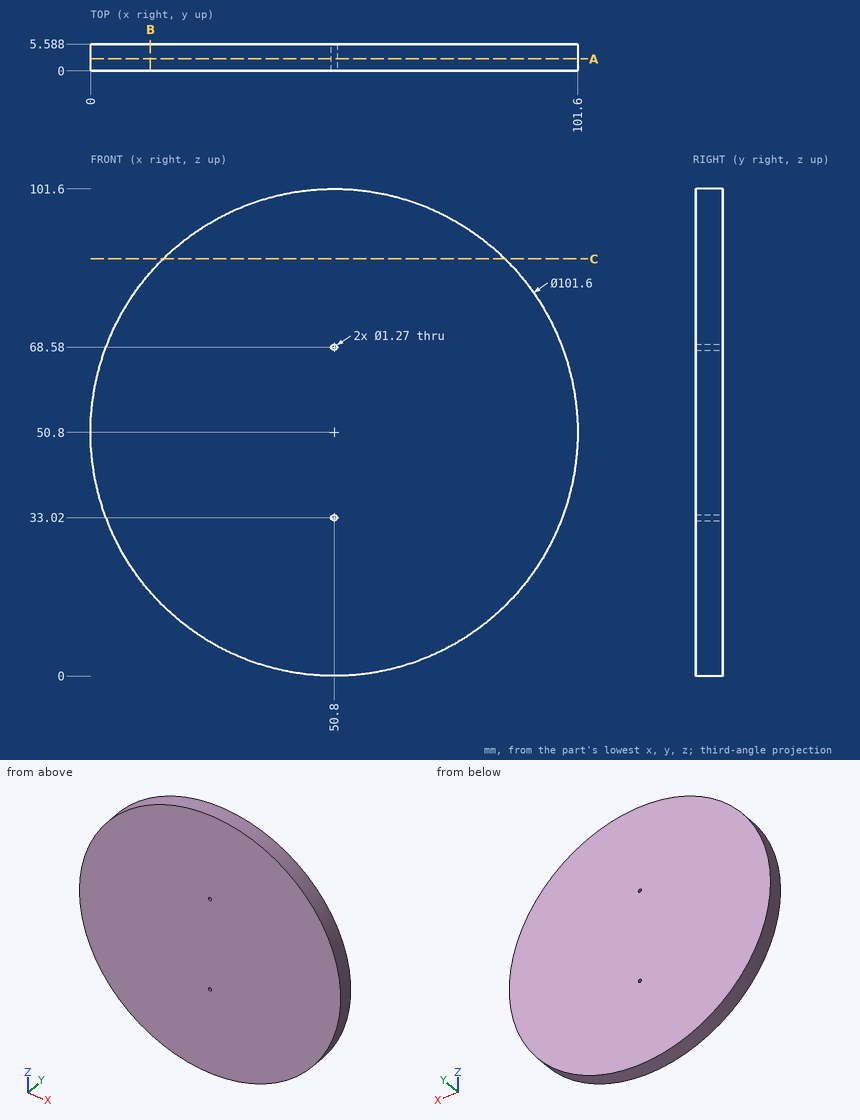
Design review of the part shown in the three views and the two pictorial views. Dimensions are in mm from the part's minimum x, y and z. Give positions to 0.01 mm unless a question says otherwise; leave off trailing zeros. Write each loop counter-clockwise with the first axis right and the second up, starting at its lowest first coordinate (ties: lowest second). Pieces come first, ordered by that corner, then holes.
(1) Wall thickness on line 1 along Z through (x, y) = (50.8, 2.95) (3 decimals); line 2 along X through (y, z) = (2.55, 68.58) (3 decimals); line 3 along Z through (x, y) = (48.5, 2.85): over which ranges is each line inside the solid? List them lowest first.
Checked values:
line 1: z = 0 to 32.385, 33.655 to 67.945, 69.215 to 101.6
line 2: x = 3.213 to 50.165, 51.435 to 98.387
line 3: z = 0.05 to 101.55
(2) Clearance check with flat-ended pins moving along their axes: pin 1 Ø3 at (y, z) = (3, 69) entering from +X; pin 2 Ø3 at (y, z) = (3, 47) entering from -X; pin 3 Ø3 at (x, y) = (44.5, 2) entering from +Z. State where each tip first meets the part, or that it passes through.
Checked values:
pin 1: stops at x = 98.78
pin 2: stops at x = 0.05
pin 3: stops at z = 101.37
(3) Add section B-B (x = 12.5). Give the boundary of the cut face in (y, z), and give its area (3 significant figures).
Checked values:
outline: (0, 17.43) - (5.59, 17.43) - (5.59, 84.17) - (0, 84.17) - close
area: 373 mm2
(4) Add section A-A (y = 2.5). Give the boundary of the cut face in (x, z) (3 decimals), and give its area (3 significant figures).
Checked values:
outline: circle Ø101.6 at (50.8, 50.8); hole circle Ø1.27 at (50.8, 33.02); hole circle Ø1.27 at (50.8, 68.58)
area: 8,100 mm2
(5) Add section C-C (z = 87). Give the boundary of the cut face in (x, y).
Checked values:
outline: (15.16, 0) - (86.44, 0) - (86.44, 5.59) - (15.16, 5.59) - close
